from build123d import *

# Parameters (mm, degrees)
F0_R     = 5.5
F1_DEPTH = 3
F2_R     = 2.8
F3_DEPTH = 5
F2_R_2   = 4.75
F2_R_3   = 4.2
F4_DEPTH = 3


with BuildPart() as f1:
    # F0 (on Right) → F1 (new body)
    with BuildSketch(Plane.YZ):
        Circle(F0_R)
    extrude(amount=F1_DEPTH)

    # F2 (on face) → F3 (join)
    with BuildSketch(Plane.YZ.offset(3)):
        Circle(F2_R)
    extrude(amount=F3_DEPTH)

    # F2 (on face) → F4 (join)
    with BuildSketch(Plane.YZ.offset(3)):
        Circle(F2_R_2)
        Circle(F2_R_3, mode=Mode.SUBTRACT)
    extrude(amount=F4_DEPTH)


solid = f1.part
Model file for the job. Use its own axes, mm. A direction names the side the tool comes from. Give positions to 0.01 mm unless a question says otherwise; leave off trailing zeros. Order: outer loops, then holes, each group sorted by start corner. A loop starts at its lowest first (then second) coordinate and runs counter-clockwise, first axis right, second up. Notation, with made-up numbers: M 89,59.5 L 109,59.5 A18 ccw 109,82.5 Z; hole C 52,69.25 d4. An arc over 180 degrees is marked long. Put each result on its own line as item: value. Start each with the question number.
(1) Band-saw the part on C-C on x = 7. Give the cut face in (y, z).
(2) Drill centre lines: L1, parallel to Z at x = 4, y = 0; L2, parallel to Y at x = 5, z = 1.75; L3, parallel to Z at x = 3.5, y = -1. Where is each one in solid material? Low to high. Write a range as [from, to].
(3) Pin check, flat tips, straight feed: pin 1 Ø2 at (x, y) = (5.5, -0.5) entering from +Z; pin 2 Ø1 at (x, y) = (2, -2.5) entering from -Z; pin 3 Ø2 at (x, y) = (4.5, -2) entering from -Z. Stop position of each tip, or through.
(4) Band-saw the part on A-A on z = 0. Give the cut face in (x, y), then the cut area to 3 significant figures.
(5) Band-saw the part on D-D on z = 3. Give the cut face in (x, y).
(6) Pull direction Y, two halves, no side cores. Call faces 3 (the face through (5.5, -2.8, 0.1)), 4 (the face through (8, 0, 0)), 5 (the face through (4.479, 4.006, 1.262)), 6 (the face through (4.479, 2.192, -4.214)): released by +Y, released by -Y, zero draft, split by the parting line, or undercut.
(7) Tool access for faces 1 (the face through (3, -5, 0)), 2 (the face through (1.48, -1.19, -5.37)): list every direction of +Z, -Z, +X, -X, +Y, -Y with a clear straight run to the whole face (end or side of a thin tool).
Results below:
1. outline: C 0,0 d5.6
2. L1: z = [-4.75, -4.2], [-2.8, 2.8], [4.2, 4.75]
2. L2: y = [-4.42, -3.82], [-2.19, 2.19], [3.82, 4.42]
2. L3: z = [-4.64, -4.08], [-2.62, 2.62], [4.08, 4.64]
3. pin 1: stops at z = 4.75
3. pin 2: stops at z = -5.12
3. pin 3: stops at z = -4.64
4. outline: M 0,-5.5 L 3,-5.5 L 3,-4.75 L 6,-4.75 L 6,-4.2 L 3,-4.2 L 3,-2.8 L 8,-2.8 L 8,2.8 L 3,2.8 L 3,4.2 L 6,4.2 L 6,4.75 L 3,4.75 L 3,5.5 L 0,5.5 Z
4. area: 64.3 mm2
5. outline: M 0,-4.61 L 3,-4.61 L 3,-3.68 L 6,-3.68 L 6,-2.94 L 3,-2.94 L 3,2.94 L 6,2.94 L 6,3.68 L 3,3.68 L 3,4.61 L 0,4.61 Z
6. face 3: undercut
6. face 4: zero draft
6. face 5: undercut
6. face 6: split by the parting line
7. face 1: +X
7. face 2: +X, -X
